```python
from build123d import *

# Parameters (mm, degrees)
SALIENTE_EXTRUIR1_DEPTH = 5
REDONDEO1_R             = 10


with BuildPart() as part:
    # Croquis1 → Saliente-Extruir1 (new body)
    with BuildSketch(Plane(origin=(0, 0, 0), x_dir=(1, 0, 0), z_dir=(0, 1, 0))):
        Polygon((0, 0), (-3, 0), (-1, 22.5), (-3, 45), (0, 45), align=None)
    extrude(amount=SALIENTE_EXTRUIR1_DEPTH)

    # Redondeo1
    redondeo1_edges = [part.edges().sort_by_distance(p)[0] for p in [
        (-1, 2.5, -22.5),
    ]]
    fillet(redondeo1_edges, radius=REDONDEO1_R)


solid = part.part
```
Check sheet for the modelled part. Datum: model origin and axes. Units: mm. A direction names the side the tool comes from. Round coordinates to 2 decimals unless told otherwise and drop trailing zeros. Order: outer loops, then holes, each group sorted by start corner. A loop starts at its lowest first (then second) coordinate and runs counter-clockwise, first axis right, second up. Notation, with made-up numbers: M 63.5,-21.75 L 106.5,-21.75 A31 ccw 106.5,7.25 Z; hole C 79,52.25 d4. An arc over 180 degrees is marked long. Answer in a Markdown table with one row per item.
(1) Section check B-B on y = 2.6. Record the boundary of the cut face in (x, z), plus the area to 3 significant figures.
Findings:
| item | result |
|---|---|
| outline | M -3,-45 L 0,-45 L 0,0 L -3,0 L -1.08,-21.61 A10 cw -1.08,-23.39 Z |
| area | 90.0 mm^2 |
(2) Draft check along Z on faces 1 (the flat face through (-0.8, 5, -22.8)), 2 (the flat face through (-2.026, 2.465, -34.041)), 3 (the flat face through (-2, 2, -45)). Enter one of: +Z half, -Z half, draft (parallel to the pull), parting line (faces both ways), or undercut.
Findings:
| item | result |
|---|---|
| face 1 | draft |
| face 2 | undercut |
| face 3 | -Z half |
(3) Section check D-D on z = -5. Record the boundary of the cut face in (x, y), plus the area to 3 significant figures.
Findings:
| item | result |
|---|---|
| outline | M -2.56,0 L 0,0 L 0,5 L -2.56,5 Z |
| area | 12.8 mm^2 |
(4) Section check C-C on z = -39. Record the boundary of the cut face in (x, y), plus the area to 3 significant figures.
Findings:
| item | result |
|---|---|
| outline | M -2.47,0 L 0,0 L 0,5 L -2.47,5 Z |
| area | 12.3 mm^2 |
(5) Section check A-A on x = -2.6. Record the boundary of the cut face in (y, z), plus the area to 3 significant figures.
Findings:
| item | result |
|---|---|
| outline | M 0,-45 L 5,-45 L 5,-40.5 L 0,-40.5 Z; M 0,-4.5 L 5,-4.5 L 5,0 L 0,0 Z |
| area | 45.0 mm^2 |
(6) Set-up check for faces 4 (the flat face through (-2.053, 2.465, -10.656)), 5 (the flat face through (0, 2, -23)): record each of +Z, -Z, +X, -X, +Y, -Y from which the full face is reachable in a straight line by a thin tool's end or side.
Findings:
| item | result |
|---|---|
| face 4 | -X, +Y, -Y |
| face 5 | +Z, -Z, +X, +Y, -Y |
(7) Material ranges on line 1 along X through (y, z) = (4.4, -41.5); line 2 along X through (y, z) = (1, -26), recorded low to high. Write a range as from..to.
Findings:
| item | result |
|---|---|
| line 1 | x = -2.69..0 |
| line 2 | x = -1.31..0 |
